For this review, take the finished solid that the model builds, in its own axes (mm). Coordinates: 2 decimals unless noted, no trailing zeros. Loops run counter-clockwise (first coordinate to the right, second up) from the corner with the lowest first, then second, coordinate; pieces in that order, holes last.
1. To check wall thickness, follow probe 1 along X at (y, z) = (-7, 72.5); probe 2 along X at (y, z) = (6, 0); probe 3 along X at (y, z) = (-10, -32). State the ranges of each line that lie inside material, in increasing order.
2. Clearance check with flat-ended pins moving along their axes: P1, Ø6, axis at x = -13, y = 4, coming from the -Z side; P2, Ø14.5, axis at x = 2, z = -54.5, coming from the +Y side; P3, Ø23.5, axis at y = -2.5, z = -53.5, coming from the -X side; P4, Ø12, axis at x = -19.5, z = -32.5, coming from the -Y side. State where each tip first meets the part, or that it passes through.
3. Take a section at A-A, the plane z = -31. State the section outline as (x, y) points.
4. Take a section at D-D, the plane y = -21. State the section outline as (x, z) points, then the cut area to 3 significant figures.
5. Take a section at C-C, the plane y = 0. State the section outline as (x, z) points, then the cut area to 3 significant figures.
6. Take a section at B-B, the plane x = 4. State the section outline as (y, z) points.
```python
from build123d import *

# Parameters (mm, degrees)
BOSS_EXTRUDE1_DEPTH     = 115
CUT_EXTRUDE1_DEPTH      = 118.660110418
CUT_EXTRUDE1_DEPTH_BACK = 118.660110418
SKETCH2_R               = 18


with BuildPart() as part:
    # Sketch1 → Boss-Extrude1 (new, symmetric)
    with BuildSketch(Plane.XY):
        Polygon((-9.009337123, 12.5), (-9.009337123, -9.009337123), (9.009337123, -9.009337123), (9.009337123, 12.5), (12.5, 12.5), (12.5, -12.5), (-12.5, -12.5), (-12.5, 12.5), align=None)
    extrude(amount=BOSS_EXTRUDE1_DEPTH, both=True)

    # Sketch2 → Cut-Extrude1 (cut, two sides: drawn at the far end of the back side and taken through both)
    with BuildSketch(Plane(origin=(0, -9.009337123, 0), x_dir=(1, 0, 0), z_dir=(0, 1, 0)).offset(-CUT_EXTRUDE1_DEPTH_BACK)):
        with Locations((8.990662877, 0)):
            Circle(SKETCH2_R)
    extrude(amount=CUT_EXTRUDE1_DEPTH + CUT_EXTRUDE1_DEPTH_BACK, mode=Mode.SUBTRACT)

    # Sketch3 → Revolve1 (revolve)
    with BuildSketch(Plane.XY.offset(115)):
        with BuildLine():
            Line((0, 32.5), (0, -32.5))
            ThreePointArc((0, -32.5), (32.5, 0), (0, 32.5))
        make_face()
    revolve1 = revolve(axis=Axis((0, 32.5, 115), (0, -1, 0)))

    # Mirror1: Revolve1 across plane
    add(revolve1.mirror(Plane.XY))


solid = part.part
```
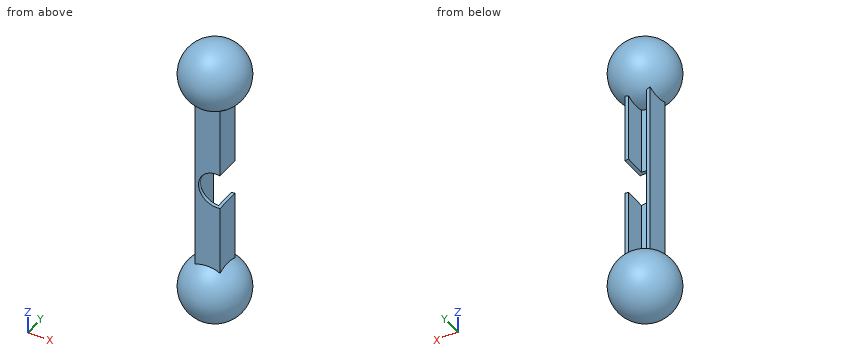
Results list:
1. probe 1: x = -12.5 to -9.01, 9.01 to 12.5
1. probe 2: x = -12.5 to -9.01
1. probe 3: x = -12.5 to 12.5
2. P1: stops at z = -145.72
2. P2: stops at y = 12.5
2. P3: stops at x = -12.5
2. P4: passes through
3. outline: (-12.5, -12.5) - (12.5, -12.5) - (12.5, 12.5) - (9.01, 12.5) - (9.01, -9.01) - (-9.01, -9.01) - (-9.01, 12.5) - (-12.5, 12.5) - close
4. outline: circle Ø49.61 at (0, -115); circle Ø49.61 at (0, 115)
4. area: 3,870 mm2
5. outline: (-12.5, -85) arc R32.5 ccw (long way) to (12.5, -85) - (12.5, -17.65) arc R18 cw to (9.01, -18) - (9.01, -83.77) arc R32.5 ccw to (-9.01, -83.77) - (-9.01, 83.77) arc R32.5 ccw to (9.01, 83.77) - (9.01, 18) arc R18 cw to (12.5, 17.65) - (12.5, 85) arc R32.5 ccw (long way) to (-12.5, 85) - close
5. area: 7,690 mm2
6. outline: (-12.5, -85.27) arc R32.25 ccw (long way) to (-9.01, -84.03) - (-9.01, -17.29) - (-12.5, -17.29) - close; (-12.5, 17.29) - (-9.01, 17.29) - (-9.01, 84.03) arc R32.25 ccw (long way) to (-12.5, 85.27) - close
